```python
from build123d import *
from OCP.BRepFilletAPI import BRepFilletAPI_MakeChamfer

# Parameters (mm, degrees)
SKETCH1_R                    = 18
BOSS_EXTRUDE1_DEPTH          = 38
SKETCH2_OUTSIDE_W            = 50.706
SKETCH2_OUTSIDE_H            = 50.706
SKETCH2_OUTSIDE_R            = 3.5
CUT_EXTRUDE1_DEPTH           = 4
SKETCH3_OUTSIDE_W            = 50.706
SKETCH3_OUTSIDE_H            = 50.706
SKETCH3_OUTSIDE_R            = 11
CUT_EXTRUDE2_DEPTH           = 9
CHAMFER1_SIZE                = 4
CHAMFER1_SIZE2               = 1.455880937
F_3_0_3_DIAMETER_HOLE1_D     = 3
F_3_0_3_DIAMETER_HOLE1_DEPTH = 34.098709071
F_3_0_3_DIAMETER_HOLE1_TIP   = 0.901290929


with BuildPart() as part:
    # Sketch1 → Boss-Extrude1 (new body)
    with BuildSketch(Plane(origin=(0, 0, 0), x_dir=(0, 0, -1), z_dir=(1, 0, 0))):
        Circle(SKETCH1_R)
    extrude(amount=BOSS_EXTRUDE1_DEPTH)

    # Sketch2 outside → Cut-Extrude1 (cut)
    with BuildSketch(Plane(origin=(38, 0, 0), x_dir=(0, 0, -1), z_dir=(1, 0, 0))):
        Rectangle(SKETCH2_OUTSIDE_W, SKETCH2_OUTSIDE_H)
        Circle(SKETCH2_OUTSIDE_R, mode=Mode.SUBTRACT)
    extrude(amount=-CUT_EXTRUDE1_DEPTH, mode=Mode.SUBTRACT)

    # Sketch3 outside → Cut-Extrude2 (cut)
    with BuildSketch(Plane.ZY):
        Rectangle(SKETCH3_OUTSIDE_W, SKETCH3_OUTSIDE_H)
        Circle(SKETCH3_OUTSIDE_R, mode=Mode.SUBTRACT)
    extrude(amount=-CUT_EXTRUDE2_DEPTH, mode=Mode.SUBTRACT)

    # Chamfer1: one chamfer whose edges measure the first distance from different faces: ONE call of the kernel's chamfer builder (chamfer() names one face for all edges)
    chamfer1_edges_1 = [part.edges().sort_by_distance(p)[0] for p in [
        (9, 0, 18),
    ]]
    chamfer1_side_1 = [part.faces().sort_by_distance(p)[0] for p in [
        (21.5, 0, 18),
    ]]
    chamfer1_edges_2 = [part.edges().sort_by_distance(p)[0] for p in [
        (0, 0, -11),
    ]]
    chamfer1_side_2 = [part.faces().sort_by_distance(p)[0] for p in [
        (4.5, 0, -11),
    ]]
    chamfer1 = BRepFilletAPI_MakeChamfer(part.part.solid().wrapped)
    for e in chamfer1_edges_1:
        chamfer1.Add(CHAMFER1_SIZE, CHAMFER1_SIZE2, e.wrapped, chamfer1_side_1[0].wrapped)  # the first distance lies on this face
    for e in chamfer1_edges_2:
        chamfer1.Add(CHAMFER1_SIZE, CHAMFER1_SIZE2, e.wrapped, chamfer1_side_2[0].wrapped)  # the first distance lies on this face
    add(Compound.cast(chamfer1.Shape()), mode=Mode.REPLACE)

    # Ø3.0 (3) Diameter Hole1
    with Locations(Plane(origin=(38, 0, 0), x_dir=(0, 0, -1), z_dir=(1, 0, 0))):
        with Locations((0, 0)):
            Hole(F_3_0_3_DIAMETER_HOLE1_D / 2, depth=F_3_0_3_DIAMETER_HOLE1_DEPTH)
            with Locations((0, 0, -(F_3_0_3_DIAMETER_HOLE1_DEPTH + F_3_0_3_DIAMETER_HOLE1_TIP / 2))):  # 118° drill point
                Cone(0, F_3_0_3_DIAMETER_HOLE1_D / 2, F_3_0_3_DIAMETER_HOLE1_TIP, mode=Mode.SUBTRACT)


solid = part.part
```
For this review, take the finished solid that the model builds, in its own axes (mm). A direction names the side the tool comes from. Coordinates: 2 decimals unless noted, no trailing zeros. Loops run counter-clockwise (first coordinate to the right, second up) from the corner with the lowest first, then second, coordinate; pieces in that order, holes last. Notation, with made-up numbers: (-10.5, -20.5) - (18.5, -20.5) arc R34 cw to (18.5, 15.5) - close; hole circle Ø6 at (12, 10). An arc over 180 degrees is marked (long way). Use one line per item in the form item = value. Start each with the question number.
1) For pin 1 (5 mm diameter, centred on x = 29, y = 4.5, fed in from +Z); pin 2 (3 mm diameter, centred on y = 14, z = -12.5, fed in from +X); pin 3 (12 mm diameter, centred on x = 6, z = 2, fed in from -Y), all flat-tipped, find the tip position at first contact; note any pin that passes through.
2) Draft analysis for pull direction Y (two halves, no side actions). For faces 4 (the face through (3, 0, 0)), 5 (the face through (34, -4, 0)), 6 (the face through (23.353, 17.847, 2.343)), state which applies: released by +Y, released by -Y, zero draft, split by the parting line, or undercut.
3) To check wall thickness, follow probe 1 along Z at (x, y) = (13, 0); probe 2 along X at (y, z) = (-11.5, -6). State the ranges of each line that lie inside material, in increasing order. Write a range as from..to.
4) For faces 1 (the face through (6.46, -10.74, -2.38)), 2 (the face through (0, 0, 0)), 3 (the face through (20.71, 0.07, -1.5)), list the 3-axis set-ups (+Z, -Z, +X, -X, +Y, -Y) from which the entire face can be reached by the end or side of a thin tool; tool diameter is ignored.
5) Take a section at B-B (x = 35). State the section outline as (y, z) points, plus the area to 3 significant figures.
6) Take a section at A-A (x = 5.5). State the section outline as (y, z) points.
From the geometry:
q1.pin_1 = 17.89
q1.pin_2 = 34
q1.pin_3 = -17.58
q2.face_4 = undercut
q2.face_5 = zero draft
q2.face_6 = split by the parting line
q3.probe_1 = -18..-1.5, 1.5..18
q3.probe_2 = 9..34
q4.face_1 = -X
q4.face_2 = +Z, -Z, -X, +Y, -Y
q4.face_3 = +X
q5.outline = circle Ø7 at (0, 0); hole circle Ø3 at (0, 0)
q5.area = 31.4 mm2
q6.outline = circle Ø22 at (0, 0); hole circle Ø3 at (0, 0)
